Verification items for the finished model (mm, model axes). A direction names the side the tool comes from. Coordinates: 2 decimals unless noted, no trailing zeros. Loops run counter-clockwise (first coordinate to the right, second up) from the corner with the lowest first, then second, coordinate; pieces in that order, holes last.
Q1. Sectioned sample at A-A (y = -6). Enter the section's corners in (x, z).
Q2. Material ranges on probe 1 along X at (y, z) = (-6, 0.9); probe 2 along Y at (x, z) = (12.5, 0.35) (3 decimals); probe 3 along Y at (x, z) = (-2.25, 1), recorded low to high.
Q3. Go/stop test with flat-tipped pins: P1, Ø0.5, axis at y = -4, z = 1, coming from the +X side; P2, Ø0.8, axis at x = -10.5, z = 1, coming from the +Y side. Record where each tip stops, or that it passes through.
Q4. Access from +Z, -Z, +X, -X, +Y, -Y to the whole of each face (thin tool, end or side, straight path). Record for faces 1 (the face through (-10.16, -4, 1)), 2 (the face through (-1.016, -4, 1)), 3 (the face through (10.6, -8.255, 0.8)), 4 (the face through (0, -30.48, 1)).
Q5. Mould release check, pull along X, two halves, no side actions. Record for faces 5 (the face through (-2.921, -4, 1)), 6 (the face through (-13, -30.48, 1)), 7 (the face through (-14.16, -20, 1)): +X half, -X half, draft (parallel to the pull), parting line (faces both ways), or undercut.
```python
from build123d import *

# Parameters (mm, degrees)
F0_W     = 28.321
F0_H     = 30.48
F1_DEPTH = 1.64
F2_W     = 1.905
F2_H     = 8.255
F2_W_2   = 1.27
F2_H_2   = 1.27
F3_DEPTH = 25
F4_R     = 0.95249
F5_SIZE  = 0.507
F6_R     = 0.63499


# Not quite as in the source:
# - a fillet or chamfer is up to 0.001 mm smaller than in the source, because OpenCascade refuses the exact size


with BuildPart() as f1:
    # F0 (on Top) → F1 (new body)
    with BuildSketch(Plane.XY):
        with Locations((0, -15.24)):
            Rectangle(F0_W, F0_H)
    extrude(amount=F1_DEPTH)

    # F2 (on Top) → F3 (cut)
    with BuildSketch(Plane.XY):
        Polygon((-10.16, 0), (-14.1605, 0), (-14.1605, -8.255), (-12.3825, -8.255), (-12.3825, -9.525), (-11.1125, -9.525), (-11.1125, -8.255), (-10.16, -8.255), align=None)
        with Locations((-1.9685, -4.1275)):
            Rectangle(F2_W, F2_H)
        Polygon((14.1605, -8.255), (14.1605, 0), (10.16, 0), (10.16, -8.255), (11.1125, -8.255), (11.1125, -9.525), (12.3825, -9.525), (12.3825, -8.255), align=None)
        with Locations((-11.7475, -29.845)):
            Rectangle(F2_W_2, F2_H_2)
        with Locations((11.7475, -29.845)):
            Rectangle(F2_W_2, F2_H_2)
    extrude(amount=F3_DEPTH, mode=Mode.SUBTRACT)

    # F4 (radius 0.9525 in the source; OpenCascade refuses exactly that, so slightly less here)
    f4_edges = [f1.edges().sort_by_distance(p)[0] for p in [
        (-2.921, -8.255, 0.82),
        (-1.016, -8.255, 0.82),
    ]]
    fillet(f4_edges, radius=F4_R)

    # F5
    f5_edges = [f1.edges().sort_by_distance(p)[0] for p in [
        (10.16, 0, 0.82),
        (-1.016, 0, 0.82),
        (-2.921, 0, 0.82),
        (-10.16, 0, 0.82),
    ]]
    chamfer(f5_edges, length=F5_SIZE)

    # F6 (radius 0.635 in the source; OpenCascade refuses exactly that, so slightly less here)
    f6_edges = [f1.edges().sort_by_distance(p)[0] for p in [
        (12.3825, -29.21, 0.82),
        (-12.3825, -29.21, 0.82),
        (-11.1125, -29.21, 0.82),
        (11.1125, -29.21, 0.82),
        (11.1125, -9.525, 0.82),
        (12.3825, -9.525, 0.82),
        (-12.3825, -9.525, 0.82),
        (-11.1125, -9.525, 0.82),
    ]]
    fillet(f6_edges, radius=F6_R)


solid = f1.part
```
Geometry check:
1. outline: (-10.16, 0) - (-2.92, 0) - (-2.92, 1.64) - (-10.16, 1.64) - close; (-1.02, 0) - (10.16, 0) - (10.16, 1.64) - (-1.02, 1.64) - close
2. probe 1: x = -10.16 to -2.92, -1.02 to 10.16
2. probe 2: y = -30.48 to -8.255
2. probe 3: y = -30.48 to -8.21
3. P1: stops at x = 10.16
3. P2: stops at y = -0.45
4. face 1: +Z, -Z, -X, +Y
4. face 2: +Z, -Z, +Y
4. face 3: +Z, -Z, +X, +Y
4. face 4: +Z, -Z, +X, -X, -Y
5. face 5: undercut
5. face 6: draft
5. face 7: -X half
